Geometry check sheet. Reference: the model listing, model coordinates, mm. A direction names the side the tool comes from. Round coordinates to 2 decimals unless told otherwise and drop trailing zeros. Loops run counter-clockwise (first coordinate to the right, second up) from the corner with the lowest first, then second, coordinate; pieces in that order, holes last. Notation, with made-up numbers: (45.25, 48.5) - (98.25, 48.5) arc R38 ccw to (98.25, 87.5) - close; hole circle Ø3 at (74.25, 4.5). An arc over 180 degrees is marked (long way). Write item = value, one per line.
```python
from build123d import *

# Parameters (mm, degrees)
SKETCH_W        = 50
SKETCH_H        = 50
PAD_DEPTH       = 10
SKETCH001_W     = 15
SKETCH001_H     = 50
PAD001_DEPTH    = 140
SKETCH004_R     = 2.6
POCKET002_DEPTH = 10
SKETCH005_R     = 8.5
SKETCH005_R_2   = 2.66237
SKETCH005_R_3   = 2.705532
POCKET_DEPTH    = 15
SKETCH006_W     = 50
SKETCH006_H     = 55
PAD002_DEPTH    = 19
SKETCH009_W     = 8
SKETCH009_H     = 50
PAD003_DEPTH    = 15
SKETCH010_R     = 8.5
POCKET003_DEPTH = 65
SKETCH011_R     = 17.1
POCKET004_DEPTH = 9
SKETCH012_R     = 2.570984
SKETCH012_R_2   = 2.587377
SKETCH012_R_3   = 2.575599
SKETCH012_R_4   = 2.613837
POCKET005_DEPTH = 65
CHAMFER_SIZE    = 7
CHAMFER001_SIZE = 7
SKETCH014_R     = 2.1
POCKET007_DEPTH = 10
SKETCH015_W     = 34
SKETCH015_H     = 5
PAD004_DEPTH    = 34
PAD005_DEPTH    = 4
PAD006_DEPTH    = 3
SKETCH018_R     = 2.1
POCKET008_DEPTH = 5
SKETCH019_W     = 50
SKETCH019_H     = 5
PAD007_DEPTH    = 25
PAD008_DEPTH    = 4
PAD009_DEPTH    = 3
SKETCH022_R     = 2.205048
SKETCH022_R_2   = 2.190785
SKETCH022_R_3   = 2.170019
SKETCH022_R_4   = 2.17643
SKETCH022_R_5   = 2.24574
POCKET009_DEPTH = 5


with BuildPart() as part:
    # Sketch → Pad (new body)
    with BuildSketch(Plane.XY):
        with Locations((0, 25)):
            Rectangle(SKETCH_W, SKETCH_H)
    extrude(amount=PAD_DEPTH)

    # Sketch001 (on Face6 of Pad) → Pad001 (join)
    with BuildSketch(Plane.XY.offset(10)):
        with Locations((0, 25)):
            Rectangle(SKETCH001_W, SKETCH001_H)
    extrude(amount=PAD001_DEPTH)

    # Sketch004 → Pocket002 (cut)
    with BuildSketch(Plane(origin=(0, 0, 0), x_dir=(1, 0, 0), z_dir=(0, 0, -1))):
        with Locations((-20, -13)):
            Circle(SKETCH004_R)
        with Locations((20, -13)):
            Circle(SKETCH004_R)
        with Locations((-20, -37)):
            Circle(SKETCH004_R)
        with Locations((20, -37)):
            Circle(SKETCH004_R)
    extrude(amount=-POCKET002_DEPTH, mode=Mode.SUBTRACT)

    # Sketch005 (on Face14 of Pocket002) → Pocket (cut)
    with BuildSketch(Plane.YZ.offset(7.5)):
        with Locations((25, 50)):
            Circle(SKETCH005_R)
        with Locations((25, 120)):
            Circle(SKETCH005_R)
        with Locations((39.142136, 64.142136)):
            Circle(SKETCH005_R_2)
        with Locations((10.857864, 35.857864)):
            Circle(SKETCH005_R_3)
    extrude(amount=-POCKET_DEPTH, mode=Mode.SUBTRACT)

    # Sketch006 (on Face13 of Pocket) → Pad002 (join)
    with BuildSketch(Plane(origin=(-7.5, 0, 0), x_dir=(0, -1, 0), z_dir=(-1, 0, 0))):
        with Locations((-25, 122.5)):
            Rectangle(SKETCH006_W, SKETCH006_H)
    extrude(amount=PAD002_DEPTH)

    # Sketch009 → Pad003 (join)
    with BuildSketch(Plane.XY.offset(10)):
        with Locations((11.5, 25)):
            Rectangle(SKETCH009_W, SKETCH009_H)
        with Locations((-11.5, 25)):
            Rectangle(SKETCH009_W, SKETCH009_H)
    extrude(amount=PAD003_DEPTH)

    # Sketch010 (on Face34 of Pad003) → Pocket003 (cut)
    with BuildSketch(Plane.YZ.offset(-7.5)):
        with Locations((25, 120)):
            Circle(SKETCH010_R)
    extrude(amount=-POCKET003_DEPTH, mode=Mode.SUBTRACT)

    # Sketch011 (on DatumPlane) → Pocket004 (cut)
    with BuildSketch(Plane(origin=(-26.5, 0, 0), x_dir=(0, -1, 0), z_dir=(-1, 0, 0))):
        with Locations((-25, 120)):
            Circle(SKETCH011_R)
    extrude(amount=-POCKET004_DEPTH, mode=Mode.SUBTRACT)

    # Sketch012 (on DatumPlane) → Pocket005 (cut)
    with BuildSketch(Plane(origin=(-26.5, 0, 0), x_dir=(0, -1, 0), z_dir=(-1, 0, 0))):
        with Locations((-39.825628, 105.174372)):
            Circle(SKETCH012_R)
        with Locations((-39.828762, 134.828762)):
            Circle(SKETCH012_R_2)
        with Locations((-10.170334, 134.829666)):
            Circle(SKETCH012_R_3)
        with Locations((-10.174481, 105.127072)):
            Circle(SKETCH012_R_4)
    extrude(amount=-POCKET005_DEPTH, mode=Mode.SUBTRACT)

    # Chamfer
    chamfer_edges = [part.edges().sort_by_distance(p)[0] for p in [
        (15.5, 25, 25),
    ]]
    chamfer(chamfer_edges, length=CHAMFER_SIZE)

    # Chamfer001
    chamfer001_edges = [part.edges().sort_by_distance(p)[0] for p in [
        (-15.5, 25, 25),
    ]]
    chamfer(chamfer001_edges, length=CHAMFER001_SIZE)

    # Sketch014 → Pocket007 (cut)
    with BuildSketch(Plane(origin=(0, 50, 0), x_dir=(-1, 0, 0), z_dir=(0, 1, 0))):
        with Locations((0, 60)):
            Circle(SKETCH014_R)
        with Locations((0, 40)):
            Circle(SKETCH014_R)
    extrude(amount=-POCKET007_DEPTH, mode=Mode.SUBTRACT)

    # Sketch015 (on DatumPlane) → Pad004 (join)
    with BuildSketch(Plane(origin=(0, 50, 0), x_dir=(-1, 0, 0), z_dir=(0, 1, 0))):
        with Locations((9.503069, 147.5)):
            Rectangle(SKETCH015_W, SKETCH015_H)
    extrude(amount=PAD004_DEPTH)

    # Sketch016 (on DatumPlane) → Pad005 (join)
    with BuildSketch(Plane.YZ.offset(7.496931)):
        Polygon((50, 145), (84, 145), (50, 130), align=None)
    extrude(amount=-PAD005_DEPTH)

    # Sketch017 (on DatumPlane) → Pad006 (join)
    with BuildSketch(Plane(origin=(-26.503069, 0, 0), x_dir=(0, -1, 0), z_dir=(-1, 0, 0))):
        Polygon((-84, 145), (-50, 145), (-50, 130), align=None)
    extrude(amount=-PAD006_DEPTH)

    # Sketch018 (on Face38 of Pad006) → Pocket008 (cut)
    with BuildSketch(Plane.XY.offset(150)):
        with Locations((-17.921772, 80.050142)):
            Circle(SKETCH018_R)
        with Locations((-17.903705, 67.549894)):
            Circle(SKETCH018_R)
        with Locations((-17.99993, 55.050264)):
            Circle(SKETCH018_R)
        with Locations((0.078158, 79.999878)):
            Circle(SKETCH018_R)
        with Locations((0.096225, 67.49963)):
            Circle(SKETCH018_R)
        with Locations((0, 55)):
            Circle(SKETCH018_R)
    extrude(amount=-POCKET008_DEPTH, mode=Mode.SUBTRACT)

    # Sketch019 (on DatumPlane) → Pad007 (join)
    with BuildSketch(Plane(origin=(-25, 0, 0), x_dir=(0, -1, 0), z_dir=(-1, 0, 0))):
        with Locations((-25, 7.5)):
            Rectangle(SKETCH019_W, SKETCH019_H)
    extrude(amount=PAD007_DEPTH)

    # Sketch020 (on DatumPlane) → Pad008 (join)
    with BuildSketch(Plane(origin=(0, 50, 0), x_dir=(-1, 0, 0), z_dir=(0, 1, 0))):
        Polygon((25, 0), (25, 5), (50, 5), align=None)
    extrude(amount=-PAD008_DEPTH)

    # Sketch021 (on DatumPlane) → Pad009 (join)
    with BuildSketch(Plane.XZ):
        Polygon((-50, 5), (-25, 5), (-25, 0), align=None)
    extrude(amount=-PAD009_DEPTH)

    # Sketch022 (on Face21 of Pad009) → Pocket009 (cut)
    with BuildSketch(Plane.XY.offset(10)):
        with Locations((-45.021925, 41.999993)):
            Circle(SKETCH022_R)
        with Locations((-45, 25)):
            Circle(SKETCH022_R_2)
        with Locations((-45, 8)):
            Circle(SKETCH022_R_3)
        with Locations((-31, 8)):
            Circle(SKETCH022_R_4)
        with Locations((-31, 25)):
            Circle(SKETCH022_R_5)
        with Locations((-31.021925, 41.999993)):
            Circle(SKETCH022_R_5)
    extrude(amount=-POCKET009_DEPTH, mode=Mode.SUBTRACT)


solid = part.part
```
(1) Section check A-A (x = 20). Enter the section's corners in (y, z), then the cut area to 3 significant figures.
Answers follow:
outline = (0, 0) - (10.4, 0) - (10.4, 10) - (0, 10) - close; (15.6, 0) - (34.4, 0) - (34.4, 10) - (15.6, 10) - close; (39.6, 0) - (50, 0) - (50, 10) - (39.6, 10) - close
area = 396 mm²
(2) Section check C-C (y = 25). State how many separate pieces and enclosed holes the cut face has, then the cut area to 3 significant figures.
Answers follow:
separate_pieces = 5
enclosed_holes = 0
area = 2,930 mm²
(3) Gauge pin test, flat ends, axial feed: pin 1 (8 mm diameter, centred on y = 10.17, z = 134.83, fed in from -X); pin 2 (3 mm diameter, centred on y = 46, z = 101, fed in from +X); pin 3 (1.5 mm diameter, centred on x = 8, z = 71.5, fed in from -Y); pin 4 (4 mm diameter, centred on y = 21.5, z = 15.5, fed in from -X). Record the tip position at first contact, or that the pin passes through.
Answers follow:
pin_1 = -26.5
pin_2 = 7.5
pin_3 = 0
pin_4 = -15.5
(4) Section check D-D (x = -31). Enter the section's corners in (y, z).
Answers follow:
outline = (0, 1.2) - (3, 1.2) - (3, 5) - (5.82, 5) - (5.82, 10) - (0, 10) - close; (10.18, 5) - (22.75, 5) - (22.75, 10) - (10.18, 10) - close; (27.25, 5) - (39.75, 5) - (39.75, 10) - (27.25, 10) - close; (44.25, 5) - (46, 5) - (46, 1.2) - (50, 1.2) - (50, 10) - (44.25, 10) - close
(5) Scan lines: L1, parallel to Y at x = 20, z = 7; L2, parallel to Y at x = -45, z = 7; L3, parallel to Y at x = -1, z = 50.5. Record each from-to range of solid material in increasing order. Write a range as [from, to].
Answers follow:
L1 = [0, 10.4], [15.6, 34.4], [39.6, 50]
L2 = [0, 5.83], [10.17, 22.81], [27.19, 39.8], [44.2, 50]
L3 = [0, 16.51], [33.49, 50]
(6) Mould release check, pull along Z, two halves, no side actions. Record for faces 4 (the cylindrical face through (-9.74, 12.21, 133.26)), 5 (the flat face through (-7.5, 25, 60)), 6 (the flat face through (7.5, 25, 87)), 7 (the flat face through (5.525, 67.238, 137.605)): pulls with the +Z half, pulls with the -Z half, needs draft (parallel to the pull), parting line crosses it, or undercut.
Answers follow:
face_4 = undercut
face_5 = undercut
face_6 = needs draft
face_7 = pulls with the -Z half
(7) Set-up check for faces 1 (the flat face through (0, 40, 60)), 2 (the flat face through (20, 25, 10)), 3 (the flat face through (-23.503, 63, 139)): record each of +Z, -Z, +X, -X, +Y, -Y from which the full face is reachable in a straight line by a thin tool's end or side.
Answers follow:
face_1 = +Y
face_2 = +Z, +X, +Y, -Y
face_3 = -Z, +Y
(8) Section check B-B (z = 117.5). Enter the section's corners in (x, y).
Answers follow:
outline = (-26.5, 0) - (7.5, 0) - (7.5, 16.88) - (-17.5, 16.88) - (-17.5, 8.08) - (-26.5, 8.08) - close; (-26.5, 41.92) - (-17.5, 41.92) - (-17.5, 33.12) - (7.5, 33.12) - (7.5, 50) - (-26.5, 50) - close
